The listing builds one solid part. Answer for the finished solid, in the listing's coordinates (mm). Face numbers are marked on the shaded views. A direction names the side the tool comes from. Give positions to 0.01 mm unless a question says otherwise; leave off trailing zeros. Order: outer loops, then holes, each group sorted by start corner. A loop starts at its lowest first (then second) coordinate and runs counter-clockwise, first axis right, second up. Notation, with made-up numbers: (4.25, -9) -> (11.25, -9) arc R30 ccw to (11.25, 30) -> close; hole circle Ø9 at (5.25, -14). An arc over 180 degrees is marked (long way). One line per question, with ' | ' between items. Start each with the question number.
```python
from build123d import *

# Parameters (mm, degrees)
F1_DEPTH     = 6.35
F2_F1_R      = 5.08
F2_F2_R      = 5.08
F3_T1_DEPTH  = 7.62
F3_T3_DEPTH  = 7.62
F3_T6_ANGLE  = 180
F3_T8_ANGLE  = 180
F3_T10_ANGLE = 180
F3_T12_ANGLE = 180


# Not quite as in the source:
# - a fillet or chamfer that OpenCascade refuses, or shapes differently, is made with other operations: its cross-section is extruded or revolved along the edge and cut away or added


with BuildPart() as f1:
    # F0 (on Top) → F1 (new body)
    with BuildSketch(Plane.XY):
        with BuildLine():
            Line((-31.75, -38.1), (31.75, -38.1))
            Line((31.75, -38.1), (31.75, -6.35))
            Line((31.75, -6.35), (82.55, -9.525))
            Line((82.55, -9.525), (82.55, 9.525))
            Line((82.55, 9.525), (31.75, 6.35))
            Line((31.75, 6.35), (31.75, 38.1))
            Line((31.75, 38.1), (-31.75, 38.1))
            Line((-31.75, 38.1), (-31.75, 31.75))
            ThreePointArc((-31.75, 31.75), (-28.575, 28.575), (-25.4, 31.75))
            Line((-25.4, 31.75), (19.05, 31.75))
            Line((19.05, 31.75), (19.05, -31.75))
            Line((19.05, -31.75), (-25.4, -31.75))
            ThreePointArc((-25.4, -31.75), (-28.575, -28.575), (-31.75, -31.75))
            Line((-31.75, -31.75), (-31.75, -38.1))
        make_face()
    extrude(amount=F1_DEPTH)

    # F2: fillet of radius 5.08 on 10 edges, made by hand

    # F2_f1
    f2_f1_edges = [f1.edges().sort_by_distance(p)[0] for p in [
        (19.05, -31.75, 3.175),
        (31.75, 6.35, 3.175),
        (31.75, -6.35, 3.175),
        (19.05, 31.75, 3.175),
    ]]
    fillet(f2_f1_edges, radius=F2_F1_R)

    # F2_f2
    f2_f2_edges = [f1.edges().sort_by_distance(p)[0] for p in [
        (31.75, -38.1, 3.175),
        (-31.75, -38.1, 3.175),
        (82.55, -9.525, 3.175),
        (82.55, 9.525, 3.175),
        (31.75, 38.1, 3.175),
        (-31.75, 38.1, 3.175),
    ]]
    fillet(f2_f2_edges, radius=F2_F2_R)

    # F3: fillet of radius 2.54 on 8 edges, made by hand

    # F3_s2 → F3_t1 (cut)
    with BuildSketch(Plane.XZ.offset(-39.37)):
        with BuildLine():
            ThreePointArc((-31.75, 3.81), (-31.0060512242, 5.6060512242), (-29.21, 6.35))
            Line((-29.21, 6.35), (-31.75, 6.35))
            Line((-31.75, 6.35), (-31.75, 3.81))
        make_face()
        with BuildLine():
            ThreePointArc((-29.21, 0), (-31.0060512242, 0.7439487758), (-31.75, 2.54))
            Line((-31.75, 2.54), (-31.75, 0))
            Line((-31.75, 0), (-29.21, 0))
        make_face()
    extrude(amount=F3_T1_DEPTH, mode=Mode.SUBTRACT)

    # F3_s4 → F3_t3 (cut)
    with BuildSketch(Plane.XZ.offset(31.75)):
        with BuildLine():
            ThreePointArc((-31.75, 3.81), (-31.0060512242, 5.6060512242), (-29.21, 6.35))
            Line((-29.21, 6.35), (-31.75, 6.35))
            Line((-31.75, 6.35), (-31.75, 3.81))
        make_face()
        with BuildLine():
            ThreePointArc((-29.21, 0), (-31.0060512242, 0.7439487758), (-31.75, 2.54))
            Line((-31.75, 2.54), (-31.75, 0))
            Line((-31.75, 0), (-29.21, 0))
        make_face()
    extrude(amount=F3_T3_DEPTH, mode=Mode.SUBTRACT)

    # F3_s5 → F3_t6 (revolve, cut)
    with BuildSketch(Plane.XZ.offset(-31.75)):
        with BuildLine():
            ThreePointArc((-31.75, 3.81), (-31.0060512242, 5.6060512242), (-29.21, 6.35))
            Line((-29.21, 6.35), (-31.75, 6.35))
            Line((-31.75, 6.35), (-31.75, 3.81))
        make_face()
    revolve(axis=Axis((-28.575, 31.75, 6.35), (0, 0, 1)), revolution_arc=F3_T6_ANGLE, mode=Mode.SUBTRACT)

    # F3_s7 → F3_t8 (revolve, cut)
    with BuildSketch(Plane.XZ.offset(-31.75)):
        with BuildLine():
            ThreePointArc((-29.21, 0), (-31.0060512242, 0.7439487758), (-31.75, 2.54))
            Line((-31.75, 2.54), (-31.75, 0))
            Line((-31.75, 0), (-29.21, 0))
        make_face()
    revolve(axis=Axis((-28.575, 31.75, 0), (0, 0, 1)), revolution_arc=F3_T8_ANGLE, mode=Mode.SUBTRACT)

    # F3_s9 → F3_t10 (revolve, cut)
    with BuildSketch(Plane.XZ.offset(31.75)):
        with BuildLine():
            ThreePointArc((-25.4, 3.81), (-26.1439487758, 5.6060512242), (-27.94, 6.35))
            Line((-27.94, 6.35), (-25.4, 6.35))
            Line((-25.4, 6.35), (-25.4, 3.81))
        make_face()
    revolve(axis=Axis((-28.575, -31.75, 6.35), (0, 0, 1)), revolution_arc=F3_T10_ANGLE, mode=Mode.SUBTRACT)

    # F3_s11 → F3_t12 (revolve, cut)
    with BuildSketch(Plane.XZ.offset(31.75)):
        with BuildLine():
            ThreePointArc((-27.94, 0), (-26.1439487758, 0.7439487758), (-25.4, 2.54))
            Line((-25.4, 2.54), (-25.4, 0))
            Line((-25.4, 0), (-27.94, 0))
        make_face()
    revolve(axis=Axis((-28.575, -31.75, 0), (0, 0, 1)), revolution_arc=F3_T12_ANGLE, mode=Mode.SUBTRACT)


solid = f1.part
```
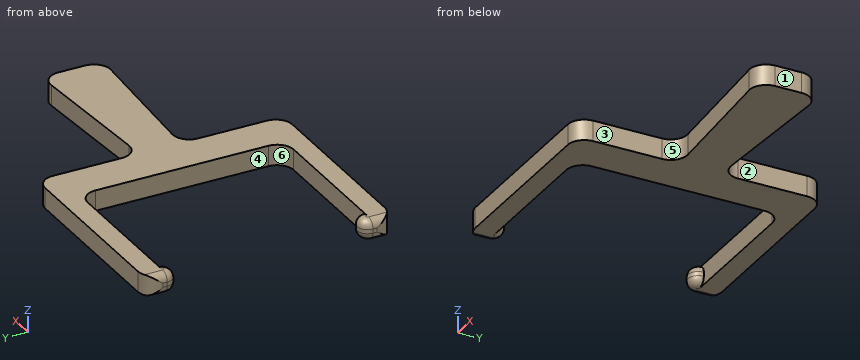
(1) Given P1, Ø1.9, axis at y = 23, z = 4, coming from the +X side; P2, Ø3, axis at y = -12.5, z = 4, coming from the -X side; P3, Ø3, axis at x = 58, z = 2, coming from the -Y side, each flat-ended and moving along its own axis, determine where each tip first touches the part or whether it passes through.
(2) Determine the mould class of the marked faces 3, 4, 5 and 6 for opening direction X: pulls with the +X half, pulls with the -X half, needs draft (parallel to the pull), parting line crosses it, or undercut.
(3) For the marked faces 1 and 2, determine the directions among +Z, -Z, +X, -X, +Y, -Y from which every point of the face is accessible in a straight line to the end or side of a thin tool.
(4) The part is cut by section B-B on y = 13. Determine the outline of the cut face in (x, z), plus the area to 3 significant figures.
(5) Consider line 1 (Y direction, x = -24.5, z = 4.25); line 2 (X direction, y = -22.5, z = 0.5); line 3 (X direction, y = -4, z = 5.5). Determine where each line is inside the solid, lowest interval first.
(6) The part is cut by section A-A on x = -10.5. Determine the outline of the cut face in (y, z), plus the area to 3 significant figures.
(7) The part is cut by section C-C on x = 50.5. Determine the outline of the cut face in (y, z), plus the area to 3 significant figures.
Result sheet:
1) P1: stops at x = 31.75 | P2: stops at x = 19.05 | P3: stops at y = -8.08
2) face 3: pulls with the +X half | face 4: pulls with the -X half | face 5: undercut | face 6: undercut
3) face 1: +Z, -Z, +X, +Y, -Y | face 2: +Z, -Z, +X, +Y
4) outline: (19.05, 0) -> (31.75, 0) -> (31.75, 6.35) -> (19.05, 6.35) -> close | area: 80.6 mm^2
5) line 1: y = -38.1 to -31.75, 31.75 to 38.1 | line 2: x = 19.05 to 31.75 | line 3: x = 19.05 to 82.55
6) outline: (-38.1, 0) -> (-31.75, 0) -> (-31.75, 6.35) -> (-38.1, 6.35) -> close; (31.75, 0) -> (38.1, 0) -> (38.1, 6.35) -> (31.75, 6.35) -> close | area: 80.6 mm^2
7) outline: (-7.52, 0) -> (7.52, 0) -> (7.52, 6.35) -> (-7.52, 6.35) -> close | area: 95.5 mm^2
